Solid Edge part; units mm, degrees
sketch "Sketch1" plane through (0, 0, 0) normal (1, 0, 0) x (0, 1, 0)
  line L0 (79.375, 10.8712) -> (0, 10.8712)
  line L1 (0, 10.8712) -> (0, 0)
  line L2 (0, 0) -> (79.375, 0)
  line L3 (79.375, 0) -> (79.375, 10.8712)
extrude "Protrusion1" add sketch "Sketch1" along normal blind 114.3
shell "Thinwall_1" thickness 3.175 removed faces 3 at (114.3, 65.3521, 1.7032) at (94.107, 0, 9.168) at (0, 65.3521, 1.7032)
sketch "Sketch2" plane through (0, 0, 0) normal (1, 0, 0) x (0, 1, 0)
  line L0 (79.375, 175.9712) -> (79.375, 10.8712)
  line L1 (79.375, 10.8712) -> (66.675, 10.8712)
  line L2 (66.675, 10.8712) -> (66.675, 175.9712)
  line L3 (66.675, 175.9712) -> (79.375, 175.9712)
extrude "Protrusion2" add sketch "Sketch2" along normal up to vertex (114.3 mm away)
hole "Hole_1" at (57.15, 66.675, 163.2712) direction (0, 1, 0) diameter 6.35 end up to next
hole "Hole1" at (57.15, 66.675, 146.2712) direction (0, 1, 0) diameter 6.35 end up to next
fillet "Round_3" radius 12.7 2 edges at (114.3, 73.025, 175.9712) (0, 73.025, 175.9712)
sketch "Sketch3" plane through (57.15, 39.6875, 0) normal (0, 0, -1) x (1, 0, 0)
  line L0 (57.15, -11.1125) -> (-57.15, -11.1125)
  line L1 (-57.15, -11.1125) -> (-57.15, 39.6875)
  line L2 (-57.15, 39.6875) -> (57.15, 39.6875)
  line L3 (57.15, 39.6875) -> (57.15, -11.1125)
extrude "Cutout1" cut sketch "Sketch3" against normal up to next
sketch "Sketch4" plane through (57.15, 39.6875, 0) normal (0, 0, -1) x (1, 0, 0)
  line L0 (25.4, 14.2875) -> (57.15, 14.2875)
  line L1 (57.15, 14.2875) -> (57.15, 39.6875)
  line L2 (57.15, 39.6875) -> (25.4, 39.6875)
  line L3 (25.4, 39.6875) -> (25.4, 14.2875)
  line L4 (-25.4, 39.6875) -> (-25.4, 14.2875)
  line L5 (-25.4, 14.2875) -> (-57.15, 14.2875)
  line L6 (-57.15, 14.2875) -> (-57.15, 39.6875)
  line L7 (-57.15, 39.6875) -> (-25.4, 39.6875)
extrude "Cutout2" cut sketch "Sketch4" against normal up to next
fillet "Round_4" radius 6.35 4 edges at (31.75, 25.4, 9.2837) (82.55, 25.4, 9.2837) (82.55, 0, 9.2837) (31.75, 0, 9.2837)
sketch "Sketch5" plane through (114.3, 52.3875, 81.6356) normal (1, 0, 0) x (0, 1, 0)
  line L0 (-26.9875, -70.7644) -> (14.2875, -29.4894)
  line L1 (14.2875, -29.4894) -> (14.2875, -70.7644)
  line L2 (14.2875, -70.7644) -> (-26.9875, -70.7644)
extrude "ExtrudedProtrusion_5" add sketch "Sketch5" against normal blind 6.35
fillet "Round_5" radius 76.2 1 edges at (111.125, 66.675, 52.1462)
mirror "Mirror1" about plane through (57.15, 0, 0) normal (-1, 0, 0) of "ExtrudedProtrusion_5"
fillet "Round1" radius 76.2 1 edges at (3.175, 66.675, 52.1462)
properties material "ABS Plastic, medium impact"
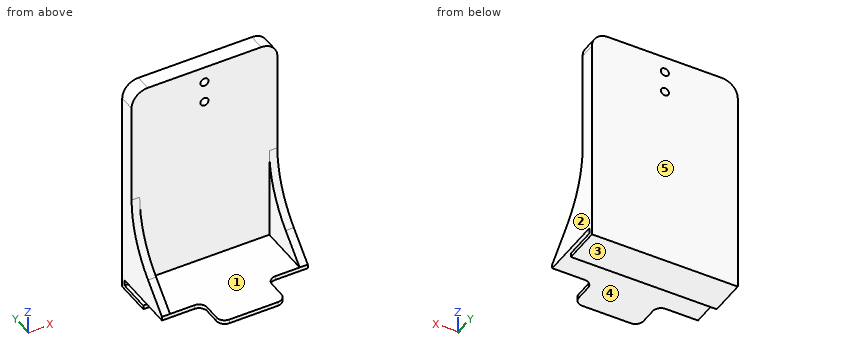
Design review of the part built by this model. Coordinates are the model's own, in mm. Face numbers are marked on the shaded views. A direction names the side the tool comes from. Coordinates: 2 decimals unless noted, no trailing zeros. Write each loop counter-clockwise with the first axis right and the second up, starting at its lowest first coordinate (ties: lowest second). Pieces come first, ordered by that corner, then holes.
1) Add section A-A (y = 71). Write out the cut boundary in (x, z) (3 decimals).
2) Add section C-C (y = 61). Write out the cut boundary in (x, z) (3 decimals), plus the area to 3 significant figures.
3) Mouldability with a two-part tool opening along Z and no side actions: class the marked faces 3, 4 and 5 as +Z half, -Z half, draft (parallel to the pull), parting line (faces both ways), or undercut.
4) Insertion check: pin 1 (12.5 mm diameter, centred on y = 55, z = 29, fed in from -X); pin 2 (12 mm diameter, centred on x = 20, y = 60, fed in from +Z); pin 3 (1 mm diameter, centred on y = 10, z = 9.5, fed in from -X); pin 4 (7.5 mm diameter, centred on x = 57.15, z = 163.27, fed in from -Y) (3 decimals). Each pin has a flat end and moves straight along its axis. Give the tip position at first contact, or say it passes through.
5) Add section B-B (x = 57.15). Write out the cut boundary in (y, z) (3 decimals), plus the area to 3 significant figures.
6) To check wall thickness, follow L1, parallel to Z at x = 57, y = 73 (3 decimals); L2, parallel to Z at x = 57.15, y = 76.75; L3, parallel to Z at x = 45.5, y = 59 (3 decimals). State the ranges of each line that lie inside material, in increasing order.
7) Machinability: for the marked faces 1 and 2, which of the approach directions +Z, -Z, +X, -X, +Y, -Y give a long, thin tool a straight path to every point of the face, cutting with its end or side? Answer none if there is none.
8) Add section D-D (x = 18). Write out the cut boundary in (y, z) (3 decimals), plus the area to 3 significant figures.
Check result:
1. outline: (0, 0) - (114.3, 0) - (114.3, 3.175) - (0, 3.175) - close; (0, 7.696) - (114.3, 7.696) - (114.3, 163.271) arc R12.7 ccw to (101.6, 175.971) - (12.7, 175.971) arc R12.7 ccw to (0, 163.271) - close; hole circle Ø6.35 at (57.15, 146.271); hole circle Ø6.35 at (57.15, 163.271)
2. outline: (0, 0) - (114.3, 0) - (114.3, 3.175) - (0, 3.175) - close; (0, 7.696) - (114.3, 7.696) - (114.3, 54.853) - (107.95, 54.853) - (107.95, 10.871) - (6.35, 10.871) - (6.35, 54.853) - (0, 54.853) - close
2. area: 1,280 mm2
3. face 3: -Z half
3. face 4: undercut
3. face 5: draft
4. pin 1: stops at x = 0
4. pin 2: stops at z = 10.87
4. pin 3: stops at x = 31.75
4. pin 4: stops at y = 66.675
5. outline: (0, 7.696) - (76.2, 7.696) - (76.2, 3.175) - (50.8, 3.175) - (50.8, 0) - (79.375, 0) - (79.375, 143.096) - (66.675, 143.096) - (66.675, 10.871) - (0, 10.871) - close; (66.675, 149.446) - (79.375, 149.446) - (79.375, 160.096) - (66.675, 160.096) - close; (66.675, 166.446) - (79.375, 166.446) - (79.375, 175.971) - (66.675, 175.971) - close
5. area: 2,290 mm2
6. L1: z = 0 to 3.175, 7.696 to 143.1, 149.443 to 160.1, 166.443 to 175.971
6. L2: z = 0 to 143.1, 149.45 to 160.1, 166.45 to 175.97
6. L3: z = 0 to 3.175, 7.696 to 10.871
7. face 1: +Z, -Y
7. face 2: +Z, -Z, +X, +Y, -Y
8. outline: (25.4, 7.696) - (76.2, 7.696) - (76.2, 3.175) - (50.8, 3.175) - (50.8, 0) - (79.375, 0) - (79.375, 175.971) - (66.675, 175.971) - (66.675, 10.871) - (25.4, 10.871) - close
8. area: 2,370 mm2
